Could you check a few things on this model? Use its own coordinates, in mm. A direction names the side the tool comes from. Coordinates: 2 decimals unless noted, no trailing zeros. Loops run counter-clockwise (first coordinate to the right, second up) from the corner with the lowest first, then second, coordinate; pieces in that order, holes last. Notation, with made-up numbers: (12, -40) -> (32, -40) arc R20 ccw to (32, -23) -> close; hole circle Ø7 at (-2, 29). An arc over 180 degrees is marked (long way). One line per question, with ' | ' between items. Start each with the question number.
(1) I'm going to push flat-ended pins straight in: pin 1 Ø1.5 at (x, z) = (-16, -74) entering from +Y; pin 2 Ø9 at (x, y) = (-56.5, 31.5) entering from +Z; pin 3 Ø24 at (x, y) = (-48.5, 38) entering from -Z (3 decimals). Where does each tip first touch, or does it pass through?
(2) Suppose I cut it at C-C (x = -44.5). Please give me the cut outline in (y, z) (3 decimals), plus the area to 3 significant figures.
(3) Suppose I cut it at A-A (y = 10). Please give me the cut outline in (x, z), plus the area to 3 significant figures.
(4) Which directions (+Z, -Z, +X, -X, +Y, -Y) give clear straight access to the entire face, cutting with the end or side of a thin tool? Please do faces 1 (the face through (-41, 23, -47)), 2 (the face through (-42, 23, -155)), 3 (the face through (-41, 13, -153)), 4 (the face through (-3, 33, -53)).
(5) If we mould it in two halves opening along Z, with no side actions, what happens to faces 5 (the face through (-41.8, 44.51, -88.34)), 6 (the face through (-43, 26, -43)), 7 (the face through (-43, 13, -3))? For each: pulls with the +Z half, pulls with the -Z half, needs draft (parallel to the pull), parting line crosses it, or undercut.
(6) If I drill on line 1 along Y through (x, z) = (-16, -47.5); line 2 along Z through (x, y) = (-34.5, 8.5); line 3 along X through (y, z) = (14, -112), over which ranges is the centre line in solid material (lowest first)?
(7) Suppose I cut it at B-B (z = -127). Please give me the cut outline in (x, y).
(8) Suppose I cut it at D-D (z = -10). Please give me the cut outline in (x, y).
Autodesk Inventor part; units mm, degrees
ref_plane "YZ Plane" through (0, 0, 0) normal (1, 0, 0) x (0, 1, 0)
ref_plane "XZ Plane" through (0, 0, 0) normal (0, 1, 0) x (-1, 0, 0)
ref_plane "XY Plane" through (0, 0, 0) normal (0, 0, 1) x (1, 0, 0)
sketch "Sketch1" plane through (0, 0, 0) normal (0, 1, 0) x (-1, 0, 0)
  line L0 (0, 0) -> (84, 0)
  line L1 (84, 0) -> (84, -156)
  line L2 (84, -156) -> (0, -156)
  line L3 (0, -156) -> (0, 0)
  line L4 (84, 0) -> (81, 0)
  line L5 (81, 0) -> (81, -3) construction
  line L6 (81, -3) -> (84, -3) construction
  line L7 (84, -3) -> (84, 0)
  line L8 (0, -156) -> (3, -156)
  line L9 (3, -156) -> (3, -153) construction
  line L10 (3, -153) -> (0, -153) construction
  line L11 (0, -153) -> (0, -156)
  line L12 (81, -3) -> (0, -3) construction
  dimension "d0" = 84
  dimension "d1" = 156
extrude "Extrusion1" add sketch "Sketch1" along normal blind 3
sketch "Sketch2" plane through (0, 3, 0) normal (0, 1, 0) x (1, 0, 0)
  line L0 (-84, 0) -> (0, 0)
  line L1 (-84, 0) -> (-42, 0)
  line L2 (-81, 3) -> (-3, 3)
  line L3 (-3, 3) -> (-3, 153)
  line L4 (-3, 153) -> (-81, 153)
  line L5 (-81, 153) -> (-81, 3)
  line L6 (-42, 0) -> (-42, 3)
  line L7 (-81, 3) -> (-47.5, 3)
  line L8 (0, 0) -> (0, 156)
  line L9 (-84, 0) -> (0, 0)
  line L10 (0, 0) -> (0, 156)
  line L11 (0, 156) -> (-84, 156)
  line L12 (-84, 156) -> (-84, 0)
  line L13 (-84, 156) -> (-84, 0)
  dimension "d12" = 42
  dimension "d13" = 78
  dimension "d14" = 150
  dimension "d15" = 3
  dimension "d16" = 33.5
extrude "Extrusion2" add sketch "Sketch2" along normal blind 20
sketch "Sketch3" plane through (0, 0, 0) normal (1, 0, 0) x (0, 0, -1)
  line L0 (156, 23) -> (0, 23)
  line L1 (0, 23) -> (90.225, 23)
  line L2 (90.225, 23) -> (90.225, 26)
  line L3 (90.225, 26) -> (0, 26)
  line L4 (0, 26) -> (0, 23)
  point P0 (0, 0)
  dimension "d19" = 90.225
  dimension "d20" = 3
extrude "Extrusion3" add sketch "Sketch3" against normal up to surface (84 mm away)
sketch "Sketch4" plane through (0, 0, 0) normal (1, 0, 0) x (0, 0, -1)
  line L0 (0, 33) -> (90.225, 44.756)
  line L1 (0, 26) -> (0, 33)
  line L2 (90.225, 23) -> (90.225, 26)
  line L3 (0, 26) -> (90.225, 26)
  line L4 (90.225, 26) -> (90.225, 44.756)
sketch "Sketch5" plane through (-84, 0, 0) normal (0, 0, 1) x (1, 0, 0)
  line L0 (3, 33) -> (3, 26)
  line L1 (3, 26) -> (81, 26)
  line L2 (81, 26) -> (81, 33)
  line L3 (81, 26) -> (3, 26)
  line L4 (3, 26) -> (3, 44.756)
  line L5 (3, 44.756) -> (81, 44.756)
  line L6 (81, 44.756) -> (81, 26)
  line L7 (3, 33) -> (81, 33)
  point P0 (84, 0)
  point P1 (84, 33)
  dimension "d27" = 3
  dimension "d28" = 78
  dimension "d29" = 7
sketch "Sketch6" plane through (0, 0, 0) normal (1, 0, 0) x (0, 0, -1)
  point P0 (0, 0)
extrude "Extrusion7" add sketch "Sketch4" against normal up to surface (84 mm away)
extrude "Extrusion10" cut sketch "Sketch5" against normal blind 87.25
properties part number "PB en arduino"
Checks:
1) pin 1: stops at y = 26 | pin 2: stops at z = -87.25 | pin 3: stops at z = -90.225
2) outline: (0, -156) -> (23, -156) -> (23, -153) -> (3, -153) -> (3, -3) -> (23, -3) -> (23, -90.225) -> (44.756, -90.225) -> (44.368, -87.25) -> (26, -87.25) -> (26, 0) -> (0, 0) -> close | area: 914 mm^2
3) outline: (-84, -156) -> (0, -156) -> (0, 0) -> (-84, 0) -> close; hole (-81, -153) -> (-3, -153) -> (-3, -3) -> (-81, -3) -> close | area: 1,400 mm^2
4) face 1: none | face 2: -Z, +X, -X, +Y | face 3: +Y | face 4: +Z, +Y
5) face 5: pulls with the +Z half | face 6: needs draft | face 7: undercut
6) line 1: y = 0 to 3, 23 to 26 | line 2: z = -156 to -153, -3 to 0 | line 3: x = -84 to -81, -3 to 0
7) outline: (-84, 0) -> (0, 0) -> (0, 23) -> (-3, 23) -> (-3, 3) -> (-81, 3) -> (-81, 23) -> (-84, 23) -> close
8) outline: (-84, 0) -> (0, 0) -> (0, 34.3) -> (-3, 34.3) -> (-3, 26) -> (-81, 26) -> (-81, 34.3) -> (-84, 34.3) -> close; hole (-81, 3) -> (-3, 3) -> (-3, 23) -> (-81, 23) -> close
